Design review of the part built by this model. Coordinates are the model's own, in mm. Face numbers are marked on the shaded views. A direction names the side the tool comes from. Give positions to 0.01 mm unless a question says otherwise; leave off trailing zeros. Order: outer loops, then holes, each group sorted by start corner. A loop starts at its lowest first (then second) coordinate and runs counter-clockwise, first axis right, second up. Notation, with made-up numbers: (-30, 0) -> (-15, 0) arc R30 cw to (-15, 33) -> close; hole circle Ø6 at (-22, -10.75). An arc over 180 degrees is marked (long way). Use a Markdown table: item, result. Add a question column.
```python
from build123d import *

# Parameters (mm, degrees)
F0_W     = 1
F0_H     = 8
F0_H_2   = 12
F0_W_2   = 16
F1_DEPTH = 0.9
F2_DEPTH = 18
F3_R     = 2
F5_DEPTH = 1
F7_DEPTH = 1


with BuildPart() as f1:
    # F0 (on Top) → F1 (new body)
    with BuildSketch(Plane.XY):
        with BuildLine():
            Line((-9, 14), (-20, 14))
            ThreePointArc((-20, 14), (-23.5355339059, 12.5355339059), (-25, 9))
            Line((-25, 9), (-25, 6))
            Line((-25, 6), (-9, 6))
            Line((-9, 6), (-9, 14))
        make_face()
        with Locations((-8.5, 10)):
            Rectangle(F0_W, F0_H)
        with Locations((-8.5, 0)):
            Rectangle(F0_W, F0_H_2)
        with Locations((-8.5, -10)):
            Rectangle(F0_W, F0_H)
        with BuildLine():
            Line((-9, -14), (-9, -6))
            Line((-9, -6), (-25, -6))
            Line((-25, -6), (-25, -9))
            ThreePointArc((-25, -9), (-23.5355339059, -12.5355339059), (-20, -14))
            Line((-20, -14), (-9, -14))
        make_face()
        with BuildLine():
            Line((25, -6), (9, -6))
            Line((9, -6), (9, -14))
            Line((9, -14), (20, -14))
            ThreePointArc((20, -14), (23.5355339059, -12.5355339059), (25, -9))
            Line((25, -9), (25, -6))
        make_face()
        with BuildLine():
            Line((20, 14), (9, 14))
            Line((9, 14), (9, 6))
            Line((9, 6), (25, 6))
            Line((25, 6), (25, 9))
            ThreePointArc((25, 9), (23.5355339059, 12.5355339059), (20, 14))
        make_face()
        with Locations((8.5, 10)):
            Rectangle(F0_W, F0_H)
        with Locations((8.5, 0)):
            Rectangle(F0_W, F0_H_2)
        with Locations((8.5, -10)):
            Rectangle(F0_W, F0_H)
        Rectangle(F0_W_2, F0_H_2)
    extrude(amount=F1_DEPTH)

    # F0 (on Top) → F2 (join)
    with BuildSketch(Plane.XY):
        with Locations((-8.5, -10)):
            Rectangle(F0_W, F0_H)
        with Locations((-8.5, 0)):
            Rectangle(F0_W, F0_H_2)
        with Locations((-8.5, 10)):
            Rectangle(F0_W, F0_H)
        with Locations((8.5, 10)):
            Rectangle(F0_W, F0_H)
        with Locations((8.5, 0)):
            Rectangle(F0_W, F0_H_2)
        with Locations((8.5, -10)):
            Rectangle(F0_W, F0_H)
    extrude(amount=F2_DEPTH)

    # F3
    f3_edges = [f1.edges().sort_by_distance(p)[0] for p in [
        (-25, 6, 0.45),
        (-9, 6, 0.45),
        (-9, -6, 0.45),
        (-25, -6, 0.45),
        (-8, 6, 0.45),
        (8, 6, 0.45),
        (25, 6, 0.45),
        (25, -6, 0.45),
        (9, 6, 0.45),
        (9, -6, 0.45),
        (8, -6, 0.45),
        (-8, -6, 0.45),
    ]]
    fillet(f3_edges, radius=F3_R)

    # F4 (on face) → F5 (join)
    with BuildSketch(Plane.YZ.offset(9)):
        Polygon((-15.4960561463, 18), (-14, 0.9), (-14, 18), align=None)
        Polygon((15.4960561463, 18), (14, 18), (14, 0.9), align=None)
    extrude(amount=-F5_DEPTH)

    # F6 (on face) → F7 (join)
    with BuildSketch(Plane(origin=(-9, 0, 0), x_dir=(0, -1, 0), z_dir=(-1, 0, 0))):
        Polygon((-14, 0.9), (-14, 18), (-15.4960561463, 18), align=None)
        Polygon((15.4960561463, 18), (14, 18), (14, 0.9), align=None)
    extrude(amount=-F7_DEPTH)


solid = f1.part
```
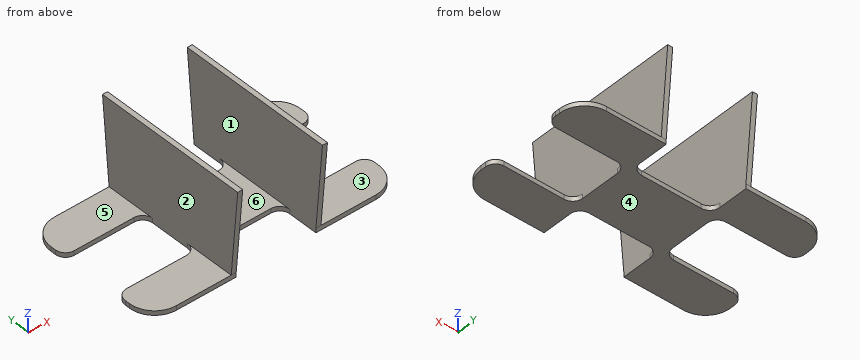
1) Insertion check: pin 1 (1.5 mm diameter, centred on x = -13.5, z = 2.5, fed in from -Y); pin 2 (0.7 mm diameter, centred on x = -17, z = 0.5, fed in from +Y); pin 3 (6 mm diameter, centred on y = 6, z = 6, fed in from +X); pin 4 (3 mm diameter, centred on x = -16.5, y = -7, fed in from +Z). Each pin has a flat end and moves straight along its axis. Give the tip position at first contact, or say it passes through.
2) The part is to be moulded in two halves that separate along X. For the marked faces 1, 2 and 3, say which applies: +X half, -X half, draft (parallel to the pull), parting line (faces both ways), or undercut.
3) Add section C-C (z = 5.75). Give the boundary of the cut face in (x, y), then the cut area to 3 significant figures.
4) Add section D-D (y = 0). Give the boundary of the cut face in (x, z).
5) Machinability: for the marked faces 4, 5 and 6, which of the approach directions +Z, -Z, +X, -X, +Y, -Y give a long, thin tool a straight path to every point of the face, cutting with its end or side? Answer none if there is none.
6) Add section B-B (y = 13). Give the boundary of the cut face in (x, z).
7) Add section A-A (x = -14). Give the boundary of the cut face in (y, z).
8) For L1, parallel to X at y = 5.5, z = 5.5; L2, parallel to Z at x = 10, y = -13.5, list the stretches that pass through material, from the lowest coordinate up. Write a range as [from, to].
Worked answers:
| question | item | result |
|---|---|---|
| 1 | pin 1 | through |
| 1 | pin 2 | y = 14 |
| 1 | pin 3 | x = 9 |
| 1 | pin 4 | z = 0.9 |
| 2 | face 1 | undercut |
| 2 | face 2 | -X half |
| 2 | face 3 | draft |
| 3 | outline | (-9, -14.42) -> (-8, -14.42) -> (-8, 14.42) -> (-9, 14.42) -> close; (8, -14.42) -> (9, -14.42) -> (9, 14.42) -> (8, 14.42) -> close |
| 3 | area | 57.7 mm^2 |
| 4 | outline | (-9, 0) -> (9, 0) -> (9, 18) -> (8, 18) -> (8, 0.9) -> (-8, 0.9) -> (-8, 18) -> (-9, 18) -> close |
| 5 | face 4 | -Z, +X, -X, +Y, -Y |
| 5 | face 5 | +Z, -X, +Y, -Y |
| 5 | face 6 | +Z, +Y, -Y |
| 6 | outline | (-23, 0) -> (-8, 0) -> (-8, 18) -> (-9, 18) -> (-9, 0.9) -> (-23, 0.9) -> close; (8, 0) -> (23, 0) -> (23, 0.9) -> (9, 0.9) -> (9, 18) -> (8, 18) -> close |
| 7 | outline | (-14, 0) -> (-6, 0) -> (-6, 0.9) -> (-14, 0.9) -> close; (6, 0) -> (14, 0) -> (14, 0.9) -> (6, 0.9) -> close |
| 8 | L1 | [-9, -8], [8, 9] |
| 8 | L2 | [0, 0.9] |
